from build123d import *

# Parameters (mm, degrees)
SKETCH1_W           = 228
SKETCH1_H           = 238.91999995
BOSS_EXTRUDE1_DEPTH = 10
SKETCH2_R           = 4.5
BOSS_EXTRUDE2_DEPTH = 10
FILLET1_R           = 5


with BuildPart() as part:
    # Sketch1 → Boss-Extrude1 (new body)
    with BuildSketch(Plane(origin=(0, 0, 0), x_dir=(0, 0, -1), z_dir=(1, 0, 0))):
        with Locations((0, 119.459999975)):
            Rectangle(SKETCH1_W, SKETCH1_H)
    extrude(amount=-BOSS_EXTRUDE1_DEPTH)

    # Sketch2 → Boss-Extrude2 (add)
    with BuildSketch(Plane(origin=(0, 0, -114), x_dir=(-1, 0, 0), z_dir=(0, 0, -1))):
        with Locations((5, 13.5)):
            Circle(SKETCH2_R)
    boss_extrude2 = extrude(amount=BOSS_EXTRUDE2_DEPTH)

    # Mirror1: Boss-Extrude2 across plane
    add(boss_extrude2.mirror(Plane.XY))

    # Fillet1
    fillet1_edges = [part.edges().sort_by_distance(p)[0] for p in [
        (-5, 238.91999995, 114),
        (-5, 238.91999995, -114),
        (-5, 0, -114),
        (-5, 0, 114),
    ]]
    fillet(fillet1_edges, radius=FILLET1_R)


solid = part.part
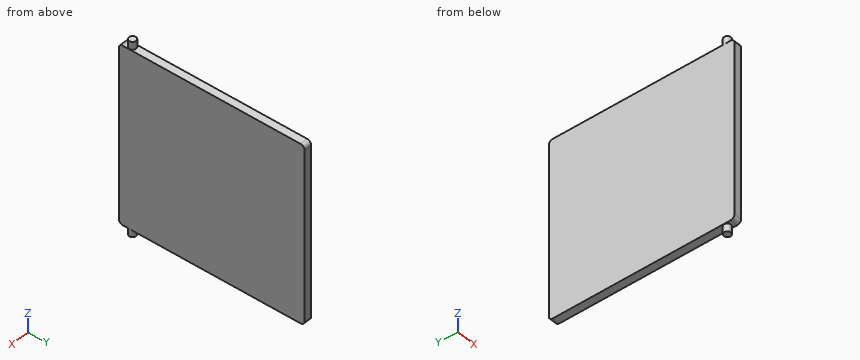
The listing builds one solid part. Answer for the finished solid, in the listing's coordinates (mm). Round coordinates to 2 decimals unless told otherwise and drop trailing zeros. Write each loop counter-clockwise with the first axis right and the second up, starting at its lowest first coordinate (ties: lowest second). Pieces come first, ordered by that corner, then holes. Notation, with made-up numbers: (-30, 51.25) - (-20, 51.25) arc R23 ccw to (-20, 71.25) - close; hole circle Ø10 at (27, 14). An arc over 180 degrees is marked (long way). Use a Markdown table: item, result. Add a question column.
1. Consider line 1 (Z direction, x = -1, y = 47). Determine where the line is inside the solid, lowest interval first.
2. The part is cut by section B-B (y = 144.5). Write down the section's boundary in (x, z), and give its area (3 significant figures).
3. The part is cut by section A-A (x = -5). Write down the section's boundary in (y, z), and give its area (3 significant figures).
4. Flat-ended cylindrical pins translate along their axes: P1, Ø8, axis at y = 65, z = 30, coming from the +X side; P2, Ø2, axis at x = -8, y = 185, coming from the +Z side. Find the tip coordinate at first contact, or state that the pin passes through.
Reported:
| question | item | result |
|---|---|---|
| 1 | line 1 | -114 to 114 |
| 2 | outline | (-10, -114) - (0, -114) - (0, 114) - (-10, 114) - close |
| 2 | area | 2,280 mm^2 |
| 3 | outline | (0, -109) arc R5 ccw to (5, -114) - (9, -114) - (9, -124) - (18, -124) - (18, -114) - (233.92, -114) arc R5 ccw to (238.92, -109) - (238.92, 109) arc R5 ccw to (233.92, 114) - (18, 114) - (18, 124) - (9, 124) - (9, 114) - (5, 114) arc R5 ccw to (0, 109) - close |
| 3 | area | 54,600 mm^2 |
| 4 | P1 | x = 0 |
| 4 | P2 | z = 114 |
